Check sheet for the modelled part. Datum: model origin and axes. Units: mm. Face numbers are marked on the shaded views. A direction names the side the tool comes from. Coordinates: 2 decimals unless noted, no trailing zeros.
1. Thickness scan on line 1 (X direction, y = 11, z = 0); line 2 (X direction, y = 7.5, z = -32); line 3 (Z direction, x = -33.5, y = 1.5). Record the ranges inside material, lowest first.
2. Gauge pin test, flat ends, axial feed: pin 1 Ø15 at (x, z) = (-31.82, -31.82) entering from +Y; pin 2 Ø1.5 at (x, y) = (-20, 6) entering from -Z; pin 3 Ø5 at (x, y) = (18, 11.5) entering from -Z; pin 4 Ø2 at (y, z) = (12, 9) entering from +X. Record the tip position at first contact, or that the pin passes through.
3. Cross-section at A-A (z = 0). Count the separate pieces of the cut face and the enclosed holes in it, then the cut area to 3 significant figures.
4. Set-up check for the marked faces 4 and 5: record each of +Z, -Z, +X, -X, +Y, -Y from which the full face is reachable in a straight line by a thin tool's end or side.
5. Draft check along Z on the marked faces 1, 2 and 3. Enter one of: released by +Z, released by -Z, zero draft, split by the parting line, or undercut.
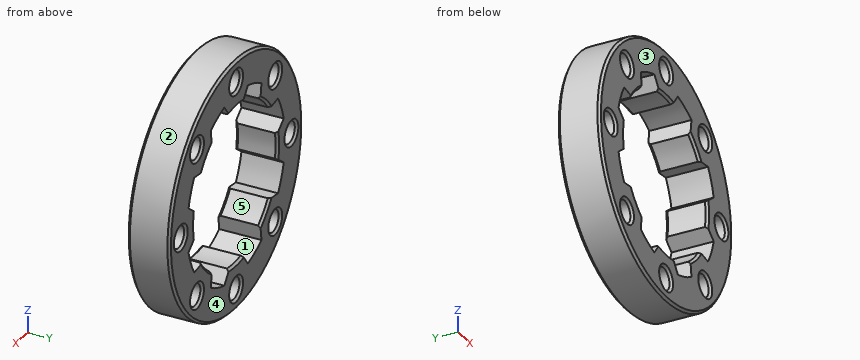
```python
from build123d import *

# Parameters (mm, degrees)
ESBO_O1_W             = 20
ESBO_O1_H             = 18
ESBO_O2_R             = 4.65
CORTE_EXTRUS_O1_DEPTH = 79.460180984
CHANFRO2_SIZE         = 1
CORTE_EXTRUS_O2_DEPTH = 79.460180984
CHANFRO3_SIZE         = 1
CHANFRO4_SIZE         = 1


with BuildPart() as part:
    # Esboço1 → Revolução1 (revolve)
    with BuildSketch(Plane.XY, mode=Mode.PRIVATE) as revolu_o1_sk:
        with Locations((44, 9)):
            Rectangle(ESBO_O1_W, ESBO_O1_H)
    revolve(revolu_o1_sk.sketch.rotate(Axis((0, -47.005255255, 0), (0, 1, 0)), 90), axis=Axis((0, -47.005255255, 0), (0, 1, 0)))

    # Esboço2 → Corte-extrusão1 (cut, through all)
    with BuildSketch(Plane(origin=(0, 18, 0), x_dir=(1, 0, 0), z_dir=(0, 1, 0))):
        with Locations(Location((-45, 0, 0), (0, 0, 270))):
            Circle(ESBO_O2_R)
        with Locations(Location((-31.819805153, 31.819805153, 0), (0, 0, 270))):
            Circle(ESBO_O2_R)
        with Locations(Location((0, 45, 0), (0, 0, 270))):
            Circle(ESBO_O2_R)
        with Locations(Location((31.819805153, 31.819805153, 0), (0, 0, 270))):
            Circle(ESBO_O2_R)
        with Locations(Location((45, 0, 0), (0, 0, 270))):
            Circle(ESBO_O2_R)
        with Locations(Location((31.819805153, -31.819805153, 0), (0, 0, 270))):
            Circle(ESBO_O2_R)
        with Locations(Location((0, -45, 0), (0, 0, 270))):
            Circle(ESBO_O2_R)
        with Locations(Location((-31.819805153, -31.819805153, 0), (0, 0, 270))):
            Circle(ESBO_O2_R)
    extrude(amount=-CORTE_EXTRUS_O1_DEPTH, mode=Mode.SUBTRACT)

    # Chanfro2
    chanfro2_edges = [part.edges().sort_by_distance(p)[0] for p in [
        (-45, 0, -4.65),
        (-45, 18, -4.65),
        (-31.819805153, 0, -36.469805153),
        (-31.819805153, 18, -36.469805153),
        (0, 0, -49.65),
        (0, 18, -49.65),
        (31.819805153, 0, -36.469805153),
        (31.819805153, 18, -36.469805153),
        (45, 0, -4.65),
        (45, 18, -4.65),
        (31.819805153, 0, 27.169805153),
        (31.819805153, 18, 27.169805153),
        (0, 0, 40.35),
        (0, 18, 40.35),
        (0, 0, 54),
        (-31.819805153, 0, 27.169805153),
        (-31.819805153, 18, 27.169805153),
        (0, 18, 54),
    ]]
    chamfer(chanfro2_edges, length=CHANFRO2_SIZE)

    # Esboço3 → Corte-extrusão2 (cut, through all)
    with BuildSketch(Plane(origin=(0, 18, 0), x_dir=(1, 0, 0), z_dir=(0, 1, 0))):
        with BuildLine():
            Line((9.547939213, 38.72951992), (5.261602172, 33.143456731))
            Line((5.261602172, 33.143456731), (19.715448431, 27.156477582))
            Line((19.715448431, 27.156477582), (20.634493603, 34.137318732))
            ThreePointArc((20.634493603, 34.137318732), (15.264890783, 36.852706357), (9.547939213, 38.72951992))
        make_face()
        with BuildLine():
            Line((27.156477582, 19.715448431), (33.143456731, 5.261602172))
            Line((33.143456731, 5.261602172), (38.72951992, 9.547939213))
            ThreePointArc((38.72951992, 9.547939213), (36.852706357, 15.264890783), (34.137318732, 20.634493603))
            Line((34.137318732, 20.634493603), (27.156477582, 19.715448431))
        make_face()
        with BuildLine():
            Line((33.143456731, -5.261602172), (27.156477582, -19.715448431))
            Line((27.156477582, -19.715448431), (34.137318732, -20.634493603))
            ThreePointArc((34.137318732, -20.634493603), (36.852706357, -15.264890783), (38.72951992, -9.547939213))
            Line((38.72951992, -9.547939213), (33.143456731, -5.261602172))
        make_face()
        with BuildLine():
            Line((19.715448431, -27.156477582), (5.261602172, -33.143456731))
            Line((5.261602172, -33.143456731), (9.547939213, -38.72951992))
            ThreePointArc((9.547939213, -38.72951992), (15.264890783, -36.852706357), (20.634493603, -34.137318732))
            Line((20.634493603, -34.137318732), (19.715448431, -27.156477582))
        make_face()
        with BuildLine():
            Line((-5.261602172, -33.143456731), (-19.715448431, -27.156477582))
            Line((-19.715448431, -27.156477582), (-20.634493603, -34.137318732))
            ThreePointArc((-20.634493603, -34.137318732), (-15.264890783, -36.852706357), (-9.547939213, -38.72951992))
            Line((-9.547939213, -38.72951992), (-5.261602172, -33.143456731))
        make_face()
        with BuildLine():
            Line((-27.156477582, -19.715448431), (-33.143456731, -5.261602172))
            Line((-33.143456731, -5.261602172), (-38.72951992, -9.547939213))
            ThreePointArc((-38.72951992, -9.547939213), (-36.852706357, -15.264890783), (-34.137318732, -20.634493603))
            Line((-34.137318732, -20.634493603), (-27.156477582, -19.715448431))
        make_face()
        with BuildLine():
            Line((-33.143456731, 5.261602172), (-27.156477582, 19.715448431))
            Line((-27.156477582, 19.715448431), (-34.137318732, 20.634493603))
            ThreePointArc((-34.137318732, 20.634493603), (-36.852706357, 15.264890783), (-38.72951992, 9.547939213))
            Line((-38.72951992, 9.547939213), (-33.143456731, 5.261602172))
        make_face()
        with BuildLine():
            Line((-19.715448431, 27.156477582), (-5.261602172, 33.143456731))
            Line((-5.261602172, 33.143456731), (-9.547939213, 38.72951992))
            ThreePointArc((-9.547939213, 38.72951992), (-15.264890783, 36.852706357), (-20.634493603, 34.137318732))
            Line((-20.634493603, 34.137318732), (-19.715448431, 27.156477582))
        make_face()
    extrude(amount=-CORTE_EXTRUS_O2_DEPTH, mode=Mode.SUBTRACT)

    # Chanfro3
    chanfro3_edges = [part.edges().sort_by_distance(p)[0] for p in [
        (0, 0, -34),
        (0, 18, -34),
        (24.04163056, 0, -24.04163056),
        (24.04163056, 18, -24.04163056),
        (34, 18, 0),
        (24.04163056, 18, 24.04163056),
        (0, 18, 34),
        (-24.04163056, 18, 24.04163056),
        (-34, 0, 0),
        (-34, 18, 0),
        (-24.04163056, 0, -24.04163056),
        (-24.04163056, 18, -24.04163056),
    ]]
    chamfer(chanfro3_edges, length=CHANFRO3_SIZE)

    # Chanfro4
    chanfro4_edges = [part.edges().sort_by_distance(p)[0] for p in [
        (34, 0, 0),
        (24.04163056, 0, 24.04163056),
        (0, 0, 34),
        (-24.04163056, 0, 24.04163056),
    ]]
    chamfer(chanfro4_edges, length=CHANFRO4_SIZE)


solid = part.part
```
Data:
1. line 1: x = -54 to -49.65, -40.35 to -34, 34 to 40.35, 49.65 to 54
1. line 2: x = -43.5 to -36.47, -27.17 to -20.35, 20.35 to 27.17, 36.47 to 43.5
1. line 3: z = -42.35 to -36.16, -27.48 to -20.55, 20.55 to 27.48, 36.16 to 42.35
2. pin 1: stops at y = 18
2. pin 2: stops at z = -50.45
2. pin 3: stops at z = -51.73
2. pin 4: stops at x = 53.4
3. separate pieces: 4
3. enclosed holes: 0
3. area: 377 mm2
4. face 4: +Z, -Z, +X, -X, +Y
4. face 5: +Y, -Y
5. face 1: undercut
5. face 2: split by the parting line
5. face 3: zero draft
